from build123d import *

# Parameters (mm, degrees)
BOSS_EXTRUDE1_DEPTH = 25.2
SKETCH2_R           = 1.6
BOSS_EXTRUDE2_DEPTH = 6
SKETCH3_W           = 19
SKETCH3_H           = 1
CUT_EXTRUDE1_DEPTH  = 38.2
CHAMFER2_SIZE       = 1.55
SKETCH4_R           = 11.1
CUT_EXTRUDE2_DEPTH  = 86.626222619
CHAMFER3_SIZE       = 1.55
CHAMFER4_SIZE       = 1
SKETCH5_R           = 1.6
CUT_EXTRUDE3_DEPTH  = 96.48869043
CHAMFER5_SIZE       = 1.55
BOSS_EXTRUDE3_START = -42
SKETCH6_W           = 20
SKETCH6_H           = 15
BOSS_EXTRUDE3_DEPTH = 3
SKETCH7_R           = 0.9
CUT_EXTRUDE4_DEPTH  = 95.097236941
CHAMFER7_SIZE       = 1.55
CHAMFER8_SIZE       = 1.55


with BuildPart() as part:
    # Sketch1 → Boss-Extrude1 (new body)
    with BuildSketch(Plane.XY):
        Polygon((0, 0), (0, 11), (-19, 11), (-19, 49.2), (8.8, 49.2), (8.8, 0), align=None)
    extrude(amount=BOSS_EXTRUDE1_DEPTH)

    # Sketch2 → Boss-Extrude2 (add)
    with BuildSketch(Plane(origin=(0, 49.2, 0), x_dir=(1, 0, 0), z_dir=(0, 1, 0))):
        Polygon((-61.5, 8.4), (-19.5, 8.4), (-19.5, 0), (8.8, 0), (8.8, -25.2), (-19.5, -25.2), (-19.5, -33.6), (-61.5, -33.6), align=None)
        with Locations(Location((-56, 2.9, 0), (0, 0, 180))):
            Circle(SKETCH2_R, mode=Mode.SUBTRACT)
        with Locations((-56, -28.1)):
            Circle(SKETCH2_R, mode=Mode.SUBTRACT)
        with Locations(Location((-25, -28.1, 0), (0, 0, 180))):
            Circle(SKETCH2_R, mode=Mode.SUBTRACT)
        with Locations((-25, 2.9)):
            Circle(SKETCH2_R, mode=Mode.SUBTRACT)
    extrude(amount=BOSS_EXTRUDE2_DEPTH)

    # Sketch3 → Cut-Extrude1 (cut)
    with BuildSketch(Plane.XZ.offset(-11)):
        with Locations((-9.5, 24.7)):
            Rectangle(SKETCH3_W, SKETCH3_H)
        with Locations((-9.5, 0.5)):
            Rectangle(SKETCH3_W, SKETCH3_H)
    extrude(amount=-CUT_EXTRUDE1_DEPTH, mode=Mode.SUBTRACT)

    # Chamfer2
    chamfer2_edges = [part.edges().sort_by_distance(p)[0] for p in [
        (-54.4, 49.2, -2.9),
        (-57.6, 49.2, 28.1),
        (-23.4, 49.2, 28.1),
        (-26.6, 49.2, -2.9),
    ]]
    chamfer(chamfer2_edges, length=CHAMFER2_SIZE)

    # Sketch4 → Cut-Extrude2 (cut, through all)
    with BuildSketch(Plane.XZ.offset(-49.2)):
        with Locations((-40.5, 12.6)):
            Circle(SKETCH4_R)
    extrude(amount=-CUT_EXTRUDE2_DEPTH, mode=Mode.SUBTRACT)

    # Chamfer3
    chamfer3_edges = [part.edges().sort_by_distance(p)[0] for p in [
        (8.8, 55.2, 12.6),
        (-61.5, 55.2, 12.6),
        (-19.5, 52.2, 0),
        (-19.5, 52.2, -8.4),
        (-61.5, 49.2, 12.6),
        (-61.5, 52.2, -8.4),
        (-61.5, 52.2, 33.6),
        (-19.5, 52.2, 33.6),
        (-19.5, 52.2, 25.2),
        (8.8, 27.6, 25.2),
        (-19, 30.1, 24.2),
        (-19, 30.1, 1),
        (8.8, 27.6, 0),
        (-51.6, 49.2, 12.6),
    ]]
    chamfer(chamfer3_edges, length=CHAMFER3_SIZE)

    # Chamfer4
    chamfer4_edges = [part.edges().sort_by_distance(p)[0] for p in [
        (0, 30.1, 24.2),
        (0, 30.1, 1),
    ]]
    chamfer(chamfer4_edges, length=CHAMFER4_SIZE - 0.0001)  # a hair under: the kernel refuses the full size

    # Sketch5 → Cut-Extrude3 (cut, through all)
    with BuildSketch(Plane(origin=(8.8, 0, 0), x_dir=(0, 0, -1), z_dir=(1, 0, 0))):
        with Locations((-5.2, 3.5)):
            Circle(SKETCH5_R)
        with Locations(Location((-20, 3.5, 0), (0, 0, 180))):
            Circle(SKETCH5_R)
    extrude(amount=-CUT_EXTRUDE3_DEPTH, mode=Mode.SUBTRACT)

    # Chamfer5
    chamfer5_edges = [part.edges().sort_by_distance(p)[0] for p in [
        (8.8, 3.5, 18.4),
        (8.8, 3.5, 6.8),
    ]]
    chamfer(chamfer5_edges, length=CHAMFER5_SIZE)

    # Sketch6 → Boss-Extrude3 (add)
    with BuildSketch(Plane.XY.offset(33.6).offset(BOSS_EXTRUDE3_START)):
        with Locations((-39, 47.7)):
            Rectangle(SKETCH6_W, SKETCH6_H)
    extrude(amount=-BOSS_EXTRUDE3_DEPTH)

    # Sketch7 → Cut-Extrude4 (cut, through all)
    with BuildSketch(Plane(origin=(0, 0, -11.4), x_dir=(-1, 0, 0), z_dir=(0, 0, -1))):
        with Locations((44, 45.2)):
            Circle(SKETCH7_R)
        with Locations((34, 45.2)):
            Circle(SKETCH7_R)
    extrude(amount=-CUT_EXTRUDE4_DEPTH, mode=Mode.SUBTRACT)

    # Chamfer7
    chamfer7_edges = [part.edges().sort_by_distance(p)[0] for p in [
        (-40.5, 55.2, 33.6),
        (-29, 55.2, -9.9),
        (-49, 55.2, -9.9),
        (-29, 52.2, -8.4),
        (-25.025, 55.2, -8.4),
        (-49, 52.2, -8.4),
        (-54.475, 55.2, -8.4),
    ]]
    chamfer(chamfer7_edges, length=CHAMFER7_SIZE)

    # Chamfer8
    chamfer8_edges = [part.edges().sort_by_distance(p)[0] for p in [
        (-39, 55.2, -11.4),
    ]]
    chamfer(chamfer8_edges, length=CHAMFER8_SIZE)


solid = part.part
Could you check a few things on this model? Use its own coordinates, in mm. A direction names the side the tool comes from. Give positions to 0.01 mm unless a question says otherwise; leave off trailing zeros. Write each loop counter-clockwise with the first axis right and the second up, starting at its lowest first coordinate (ties: lowest second). Pieces come first, ordered by that corner, then holes. Notation, with made-up numbers: (18, 26) -> (46, 26) arc R22 cw to (46, 65) -> close; hole circle Ø4 at (33, 82). An arc over 180 degrees is marked (long way). Answer as CSV lines item,"result". Start each with the question number.
(1) Please list where these lines run through material, in increasing order: line 1 (Z direction, x = -25, y = 53); line 2 (X direction, y = 52, z = 28); line 3 (Y direction, x = 1.5, z = 5.2).
(2) Which directions (+Z, -Z, +X, -X, +Y, -Y) give clear straight access to the entire face, cutting with the end or side of a thin tool? Please do faces 5 (the face through (-9, 11, 12)), 6 (the face through (-39, 45, -8.4)), 7 (the face through (-39.14, 54.44, -10.61)).
(3) I'm going to push flat-ended pins straight in: pin 1 Ø10 at (y, z) = (33, 11) entering from -X; pin 2 Ø1.6 at (y, z) = (51, -5.5) entering from +X; pin 3 Ø5.5 at (x, z) = (-11, 16.5) entering from -Y. Where does each tip first touch, or does it pass through?
(4) If we section it at D-D, the plane y = 45.2: Give the number of separate pieces and of enclosed holes in the cut face, and give its area (3 significant figures).
(5) If we section it at A-A, the plane z = -2.9: Write out the boundary of the cut face in (x, y).
(6) If we mould it in two halves opening along X, with no side actions, what happens to faces 1 (the face through (-27, 55.2, 11)), 2 (the face through (-18.71, 52.16, 25.96)), 3 (the face through (-43.34, 45.81, -9.92)), 4 (the face through (-51.59, 52.94, 13.09))? For each: +X half, -X half, draft (parallel to the pull), parting line (faces both ways), or undercut.
(7) If we section it at C-C, the plane x = -25: Write out the boundary of the cut face in (y, z), and give its area (3 significant figures).
Answer list:
1,line 1,"-8.4 to -4.5, -1.3 to 26.5, 29.7 to 33.6"
1,line 2,"-61.5 to -57.6, -54.4 to -26.6, -23.4 to -19.5"
1,line 3,"0 to 1.9, 5.1 to 55.2"
2,face 5,"+Z, -Z, -X, -Y"
2,face 6,"+Z, +X, -X, -Y"
2,face 7,"-Z, +X, -X, +Y"
3,pin 1,"x = -19"
3,pin 2,"x = -19.5"
3,pin 3,"y = 11"
4,separate pieces,"4"
4,enclosed holes,"0"
4,area,"708 mm^2"
5,outline,"(-61.5, 50.75) -> (-59.95, 49.2) -> (-59.15, 49.2) -> (-57.6, 50.75) -> (-57.6, 55.2) -> (-59.95, 55.2) -> (-61.5, 53.65) -> close; (-54.4, 50.75) -> (-52.85, 49.2) -> (-28.15, 49.2) -> (-26.6, 50.75) -> (-26.6, 55.2) -> (-54.4, 55.2) -> close; (-23.4, 50.75) -> (-21.85, 49.2) -> (-19.5, 49.2) -> (-19.5, 55.2) -> (-23.4, 55.2) -> close"
6,face 1,"draft"
6,face 2,"+X half"
6,face 3,"undercut"
6,face 4,"undercut"
7,outline,"(49.2, -8.4) -> (53.65, -8.4) -> (55.2, -6.85) -> (55.2, -4.5) -> (50.75, -4.5) -> (49.2, -6.05) -> close; (49.2, 0.25) -> (50.75, -1.3) -> (55.2, -1.3) -> (55.2, 26.5) -> (50.75, 26.5) -> (49.2, 24.95) -> close; (49.2, 31.25) -> (50.75, 29.7) -> (55.2, 29.7) -> (55.2, 32.05) -> (53.65, 33.6) -> (49.2, 33.6) -> close"
7,area,"206 mm^2"
